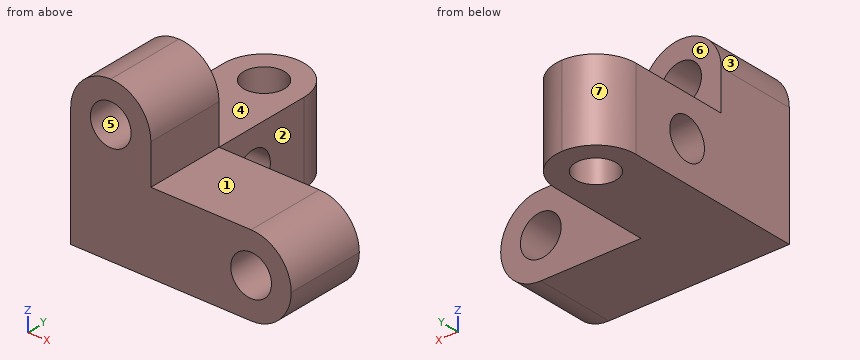
```python
from build123d import *

# Parameters (mm, degrees)
SKETCH1_W           = 33
SKETCH1_H           = 24
BOSS_EXTRUDE1_DEPTH = 33
SKETCH2_W           = 21
SKETCH2_H           = 21
CUT_EXTRUDE1_DEPTH  = 53.478567054
SKETCH3_W           = 21
SKETCH3_H           = 12
CUT_EXTRUDE2_DEPTH  = 53.478567054
SKETCH4_W           = 12
SKETCH4_H           = 21
CUT_EXTRUDE3_DEPTH  = 53.478567054
SKETCH5_R           = 3.05
CUT_EXTRUDE4_DEPTH  = 53.478567054
SKETCH6_R           = 3.05
CUT_EXTRUDE5_DEPTH  = 53.478567054
SKETCH7_R           = 3.05
CUT_EXTRUDE6_DEPTH  = 53.478567054
FILLET1_R           = 6


with BuildPart() as part:
    # Sketch1 → Boss-Extrude1 (new body)
    with BuildSketch(Plane(origin=(0, 0, 0), x_dir=(1, 0, 0), z_dir=(0, 1, 0))):
        with Locations((16.5, -12)):
            Rectangle(SKETCH1_W, SKETCH1_H)
    extrude(amount=BOSS_EXTRUDE1_DEPTH)

    # Sketch2 → Cut-Extrude1 (cut, through all)
    with BuildSketch(Plane.XY.offset(24)):
        with Locations((22.5, 22.5)):
            Rectangle(SKETCH2_W, SKETCH2_H)
    extrude(amount=-CUT_EXTRUDE1_DEPTH, mode=Mode.SUBTRACT)

    # Sketch3 → Cut-Extrude2 (cut, through all)
    with BuildSketch(Plane.XZ):
        with Locations((22.5, 18)):
            Rectangle(SKETCH3_W, SKETCH3_H)
    extrude(amount=-CUT_EXTRUDE2_DEPTH, mode=Mode.SUBTRACT)

    # Sketch4 → Cut-Extrude3 (cut, through all)
    with BuildSketch(Plane.ZY):
        with Locations((18, 22.5)):
            Rectangle(SKETCH4_W, SKETCH4_H)
    extrude(amount=-CUT_EXTRUDE3_DEPTH, mode=Mode.SUBTRACT)

    # Sketch5 → Cut-Extrude4 (cut, through all)
    with BuildSketch(Plane.ZY):
        with Locations((6, 18)):
            Circle(SKETCH5_R)
    extrude(amount=-CUT_EXTRUDE4_DEPTH, mode=Mode.SUBTRACT)

    # Sketch6 → Cut-Extrude5 (cut, through all)
    with BuildSketch(Plane.XZ):
        with Locations(Location((6, 18, 0), (0, 0, 270))):
            Circle(SKETCH6_R)
        with Locations(Location((27, 6, 0), (0, 0, 270))):
            Circle(SKETCH6_R)
    extrude(amount=-CUT_EXTRUDE5_DEPTH, mode=Mode.SUBTRACT)

    # Sketch7 → Cut-Extrude6 (cut, through all)
    with BuildSketch(Plane(origin=(0, 0, 0), x_dir=(-1, 0, 0), z_dir=(0, 0, -1))):
        with Locations((-6, 27)):
            Circle(SKETCH7_R)
    extrude(amount=-CUT_EXTRUDE6_DEPTH, mode=Mode.SUBTRACT)

    # Fillet1
    fillet1_edges = [part.edges().sort_by_distance(p)[0] for p in [
        (12, 33, 6),
        (0, 33, 6),
        (33, 6, 0),
        (33, 6, 12),
        (0, 6, 24),
        (12, 6, 24),
    ]]
    fillet(fillet1_edges, radius=FILLET1_R - 0.0001)  # a hair under: the kernel refuses the full size


solid = part.part
```
For this review, take the finished solid that the model builds, in its own axes (mm). Face numbers are marked on the shaded views. A direction names the side the tool comes from. Coordinates: 2 decimals unless noted, no trailing zeros. Write each loop counter-clockwise with the first axis right and the second up, starting at its lowest first coordinate (ties: lowest second). Pieces come first, ordered by that corner, then holes.
(1) Tool access review of the marked faces 1, 2, 3 and 4: name each direction out of +Z, -Z, +X, -X, +Y, -Y from which nothing blocks a thin tool from reaching the whole face with its end or side.
(2) Wall thickness on probe 1 along X at (y, z) = (8.5, 6); probe 2 along Y at (x, z) = (5, 5.25); probe 3 along X at (y, z) = (5, 18): over which ranges is each line inside the solid? List them lowest first.
(3) Add section D-D on x = 8. Give the boundary of the cut face in (y, z), then the cut area to 3 significant figures.
(4) The part is to be moulded in two halves that separate along X. For the marked faces 5, 6 and 7, say which applies: +X half, -X half, draft (parallel to the pull), parting line (faces both ways), or undercut.
(5) For pin 1 Ø9.5 at (x, z) = (18, 6) entering from +Y; pin 2 Ø3 at (y, z) = (5.5, 15) entering from +X; pin 3 Ø5 at (x, y) = (16.5, 24) entering from -Z; pin 4 Ø6 at (x, y) = (14.5, 19) entering from +Z, all flat-tipped, find the tip position at first contact; note any pin that passes through.
(6) Add section B-B on y = 18. Give the boundary of the cut face in (x, z).
(7) Add section A-A on y = 6. Count the separate pieces of the cut face and the enclosed holes in it, then the cut area to 3 significant figures.
Answer sheet:
1. face 1: +Z, +X, +Y, -Y
1. face 2: +Z, -Z, +X, +Y
1. face 3: +Z, -X, +Y, -Y
1. face 4: +Z, +X, -X, +Y
2. probe 1: x = 0 to 23.95, 30.05 to 33
2. probe 2: y = 0 to 15.04, 20.96 to 24.12, 29.88 to 32.92
2. probe 3: x = 0 to 2.95, 9.05 to 12
3. outline: (0, 0) - (24.7, 0) - (24.7, 12) - (12, 12) - (12, 15.7) - (0, 15.7) - close; (0, 20.3) - (12, 20.3) - (12, 23.66) - (0, 23.66) - close; (29.3, 0) - (32.66, 0) - (32.66, 12) - (29.3, 12) - close; hole circle Ø6.1 at (18, 6)
3. area: 392 mm2
4. face 5: undercut
4. face 6: draft
4. face 7: -X half
5. pin 1: stops at y = 12
5. pin 2: stops at x = 12
5. pin 3: passes through
5. pin 4: stops at z = 12
6. outline: (0, 0) - (12, 0) - (12, 2.95) - (0, 2.95) - close; (0, 9.05) - (12, 9.05) - (12, 12) - (0, 12) - close
7. separate pieces: 1
7. enclosed holes: 2
7. area: 451 mm2
